Here's how the part is built. I have some questions about the finished solid (model axes, mm). Face numbers are marked on the shaded views. A direction names the side the tool comes from. Give positions to 0.01 mm unless a question says otherwise; leave off trailing zeros. Loops run counter-clockwise (first coordinate to the right, second up) from the corner with the lowest first, then second, coordinate; pieces in that order, holes last.
Q1. Thinking about a two-plate mould opening in X: for the marked faces 1, 2 and 3, which applies, pulls with the +X half, pulls with the -X half, needs draft (parallel to the pull), parting line crosses it, or undercut?
Q2. Suppose I cut it at B-B (x = -24). List the corners of the cut face in (y, z) for me, and give its area (3 significant figures).
Q3. I need wall thicknesses on probe 1 along X at (y, z) = (-11.5, 120); probe 2 along Y at (x, z) = (-76, 101.5); probe 3 along X at (y, z) = (-42.5, 92). Which ranges of each line are inside material? Lowest first, please.
Q4. Suppose I cut it at C-C (y = -19.5). List the corners of the cut face in (x, z) for me.
Q5. Suppose I cut it at A-A (z = 108). List the corners of the cut face in (x, y) for me, and give its area (3 significant figures).
Q6. I'm going to push flat-ended pins straight in: P1, Ø5, axis at x = -58.63, y = 31.73, coming from the +Z side; P2, Ø6, axis at y = -11.5, z = 111.5, coming from the +X side; P3, Ø3.5, axis at y = -46, z = 99.5, coming from the -X side; P4, Ø1.2, axis at x = 14.5, y = 51, coming from the +Z side. Where does each tip first touch, or does it pass through?
Q7. Suppose I cut it at D-D (z = 118). List the corners of the cut face in (x, y) for me, and give its area (3 significant figures).
Q8. For the marked faces 4 and 5, which set-ups out of +Z, -Z, +X, -X, +Y, -Y let a thin tool reach every point of the face, with its end or its side?
```python
from build123d import *

# Parameters (mm, degrees)
SCHIZZO1_W                        = 100.974800609
SCHIZZO1_H                        = 100.97480061
ESTRUSIONE_ESTRUSIONE1_DEPTH      = 3
SCHIZZO3_R                        = 2
TAGLIO_ESTRUSIONE1_DEPTH          = 10
RACCORDO1_R                       = 4
TAGLIO_ESTRUSIONE2_DEPTH          = 3
ESTRUSIONE_ESTRUSIONE2_DEPTH      = 32
ESTRUSIONE_ESTRUSIONE2_DEPTH_BACK = 3
ESTRUSIONE_ESTRUSIONE3_START      = 3
ESTRUSIONE_ESTRUSIONE3_DEPTH      = 3
TAGLIO_ESTRUSIONE3_REACH          = 187.694
SCHIZZO7_W                        = 16.242748833
SCHIZZO7_H                        = 14.432058418
SCHIZZO7_W_2                      = 64.496064987
SCHIZZO7_H_2                      = 15.3
TAGLIO_ESTRUSIONE4_REACH          = 177.413
SCHIZZO8_W                        = 15.4
SCHIZZO8_H                        = 29.105346697
SMUSSO1_SIZE                      = 3
SCHIZZO9_R                        = 2
SCHIZZO9_R_2                      = 1.85551968
TAGLIO_ESTRUSIONE5_DEPTH          = 108.867451135
SCHIZZO10_R                       = 1.6
TAGLIO_ESTRUSIONE6_DEPTH          = 5


with BuildPart() as part:
    # Schizzo1 → Estrusione-Estrusione1 (new body)
    with BuildSketch(Plane(origin=(0, 0, 94.00326253), x_dir=(-1, 0, 0), z_dir=(0, 0, -1))):
        with Locations((31.141269188, 5.2439824)):
            Rectangle(SCHIZZO1_W, SCHIZZO1_H)
    extrude(amount=ESTRUSIONE_ESTRUSIONE1_DEPTH)

    # Schizzo3 → Taglio-Estrusione1 (cut)
    with BuildSketch(Plane.XY.offset(94.00326253)):
        with Locations((-77.128669492, 51.231382705)):
            Circle(SCHIZZO3_R)
        with Locations((14.871330508, 51.231382705)):
            Circle(SCHIZZO3_R)
        with Locations((-77.128669492, -40.768617295)):
            Circle(SCHIZZO3_R)
        with Locations((14.871330508, -40.768617295)):
            Circle(SCHIZZO3_R)
    extrude(amount=-TAGLIO_ESTRUSIONE1_DEPTH, mode=Mode.SUBTRACT)

    # Raccordo1
    raccordo1_edges = [part.edges().sort_by_distance(p)[0] for p in [
        (19.346131117, 55.731382705, 92.50326253),
        (-81.628669492, 55.731382705, 92.50326253),
        (-81.628669492, -45.243417905, 92.50326253),
        (19.346131117, -45.243417905, 92.50326253),
    ]]
    fillet(raccordo1_edges, radius=RACCORDO1_R)

    # Schizzo4 → Taglio-Estrusione2 (cut)
    with BuildSketch(Plane.XY.offset(94.00326253)):
        with BuildLine():
            Line((-74.872857768, -44.07184503), (12.615518783, -44.07184503))
            ThreePointArc((12.615518783, -44.07184503), (12.042903383, -37.940190171), (18.174558242, -38.512805571))
            Line((18.174558242, -38.512805571), (18.174558242, 48.97557098))
            ThreePointArc((18.174558242, 48.97557098), (12.027018614, 48.418930065), (12.652868681, 54.559809829))
            Line((12.652868681, 54.559809829), (-74.910207666, 54.559809829))
            ThreePointArc((-74.910207666, 54.559809829), (-74.300242368, 48.40295558), (-80.457096617, 49.012920878))
            Line((-80.457096617, 49.012920878), (-80.457096617, -38.550155469))
            ThreePointArc((-80.457096617, -38.550155469), (-74.316216853, -37.924305402), (-74.872857768, -44.07184503))
        make_face()
    extrude(amount=-TAGLIO_ESTRUSIONE2_DEPTH, mode=Mode.SUBTRACT)

    # Schizzo5 → Estrusione-Estrusione2 (add, two sides: drawn at the far end of the back side and taken through both)
    with BuildSketch(Plane.XY.offset(94.00326253).offset(-ESTRUSIONE_ESTRUSIONE2_DEPTH_BACK)):
        with BuildLine():
            Line((-77.628669492, 58.731382705), (15.346131117, 58.731382705))
            ThreePointArc((15.346131117, 58.731382705), (20.295878585, 56.681130173), (22.346131117, 51.731382705))
            Line((22.346131117, 51.731382705), (22.346131117, -41.243417905))
            ThreePointArc((22.346131117, -41.243417905), (20.295878585, -46.193165373), (15.346131117, -48.243417905))
            Line((15.346131117, -48.243417905), (-77.628669492, -48.243417905))
            ThreePointArc((-77.628669492, -48.243417905), (-82.578416961, -46.193165373), (-84.628669492, -41.243417905))
            Line((-84.628669492, -41.243417905), (-84.628669492, 51.731382705))
            ThreePointArc((-84.628669492, 51.731382705), (-82.578416961, 56.681130173), (-77.628669492, 58.731382705))
        make_face()
        with BuildLine():
            Line((-77.628669492, 55.731382705), (15.346131117, 55.731382705))
            ThreePointArc((15.346131117, 55.731382705), (18.174558242, 54.559809829), (19.346131117, 51.731382705))
            Line((19.346131117, 51.731382705), (19.346131117, -41.243417905))
            ThreePointArc((19.346131117, -41.243417905), (18.174558242, -44.07184503), (15.346131117, -45.243417905))
            Line((15.346131117, -45.243417905), (-77.628669492, -45.243417905))
            ThreePointArc((-77.628669492, -45.243417905), (-80.457096617, -44.07184503), (-81.628669492, -41.243417905))
            Line((-81.628669492, -41.243417905), (-81.628669492, 51.731382705))
            ThreePointArc((-81.628669492, 51.731382705), (-80.457096617, 54.559809829), (-77.628669492, 55.731382705))
        make_face(mode=Mode.SUBTRACT)
    extrude(amount=ESTRUSIONE_ESTRUSIONE2_DEPTH + ESTRUSIONE_ESTRUSIONE2_DEPTH_BACK)

    # Schizzo6 → Estrusione-Estrusione3 (add)
    with BuildSketch(Plane(origin=(0, 0, 91.00326253), x_dir=(-1, 0, 0), z_dir=(0, 0, -1)).offset(ESTRUSIONE_ESTRUSIONE3_START)):
        with BuildLine():
            Line((-15.346131117, 58.731382705), (77.628669492, 58.731382705))
            ThreePointArc((77.628669492, 58.731382705), (82.578416961, 56.681130173), (84.628669492, 51.731382705))
            Line((84.628669492, 51.731382705), (84.628669492, -41.243417905))
            ThreePointArc((84.628669492, -41.243417905), (82.578416961, -46.193165373), (77.628669492, -48.243417905))
            Line((77.628669492, -48.243417905), (-15.346131117, -48.243417905))
            ThreePointArc((-15.346131117, -48.243417905), (-20.295878585, -46.193165373), (-22.346131117, -41.243417905))
            Line((-22.346131117, -41.243417905), (-22.346131117, 51.731382705))
            ThreePointArc((-22.346131117, 51.731382705), (-20.295878585, 56.681130173), (-15.346131117, 58.731382705))
        make_face()
    extrude(amount=-ESTRUSIONE_ESTRUSIONE3_DEPTH)

    # Schizzo7 → Taglio-Estrusione3 (cut, up to next)
    with BuildSketch(Plane.XZ.offset(48.243417905), mode=Mode.PRIVATE) as taglio_estrusione3_sk1:
        with Locations((2.075800916, 102.505448711)):
            Rectangle(SCHIZZO7_W, SCHIZZO7_H)
    taglio_estrusione3_tool1 = extrude(taglio_estrusione3_sk1.sketch, amount=-TAGLIO_ESTRUSIONE3_REACH, mode=Mode.PRIVATE) & part.part
    # Schizzo7 → Taglio-Estrusione3 (cut, up to next)
    with BuildSketch(Plane.XZ.offset(48.243417905), mode=Mode.PRIVATE) as taglio_estrusione3_sk2:
        with Locations((-40.245307891, 103.027287944)):
            Rectangle(SCHIZZO7_W_2, SCHIZZO7_H_2)
    taglio_estrusione3_tool2 = extrude(taglio_estrusione3_sk2.sketch, amount=-TAGLIO_ESTRUSIONE3_REACH, mode=Mode.PRIVATE) & part.part
    add(taglio_estrusione3_tool1.solids().sort_by_distance((2.075801, -48.243418, 102.505449))[0], mode=Mode.SUBTRACT)
    add(taglio_estrusione3_tool2.solids().sort_by_distance((-40.245308, -48.243418, 103.027288))[0], mode=Mode.SUBTRACT)

    # Schizzo8 → Taglio-Estrusione4 (cut, up to next)
    with BuildSketch(Plane(origin=(22.346131117, 0, 0), x_dir=(0, 0, -1), z_dir=(1, 0, 0)), mode=Mode.PRIVATE) as taglio_estrusione4_sk1:
        with Locations((-106.101551061, -6.264379468)):
            Rectangle(SCHIZZO8_W, SCHIZZO8_H)
    taglio_estrusione4_tool1 = extrude(taglio_estrusione4_sk1.sketch, amount=-TAGLIO_ESTRUSIONE4_REACH, mode=Mode.PRIVATE) & part.part
    add(taglio_estrusione4_tool1.solids().sort_by_distance((22.346131, -6.264379, 106.101551))[0], mode=Mode.SUBTRACT)

    # Smusso1
    smusso1_edges = [part.edges().sort_by_distance(p)[0] for p in [
        (2.075800916, -48.243417905, 95.289419502),
    ]]
    chamfer(smusso1_edges, length=SMUSSO1_SIZE - 0.0001)  # a hair under: the kernel refuses the full size

    # Schizzo9 → Taglio-Estrusione5 (cut, through all)
    with BuildSketch(Plane.XY.offset(94.00326253)):
        with Locations((-77.128669492, 51.231382705)):
            Circle(SCHIZZO9_R)
        with Locations((14.871330508, 51.231382705)):
            Circle(SCHIZZO9_R_2)
        with Locations((14.871330508, -40.768617295)):
            Circle(SCHIZZO9_R)
        with Locations((-77.128669492, -40.768617295)):
            Circle(SCHIZZO9_R)
    extrude(amount=-TAGLIO_ESTRUSIONE5_DEPTH, mode=Mode.SUBTRACT)

    # Schizzo10 → Taglio-Estrusione6 (cut)
    with BuildSketch(Plane(origin=(0, 0, 88.00326253), x_dir=(-1, 0, 0), z_dir=(0, 0, -1))):
        with Locations((3.653868883, 31.731382705)):
            Circle(SCHIZZO10_R)
        with Locations((3.653868883, -14.268617295)):
            Circle(SCHIZZO10_R)
        with Locations((58.628669492, -14.268617295)):
            Circle(SCHIZZO10_R)
        with Locations((58.628669492, 31.731382705)):
            Circle(SCHIZZO10_R)
    extrude(amount=-TAGLIO_ESTRUSIONE6_DEPTH, mode=Mode.SUBTRACT)


solid = part.part
```
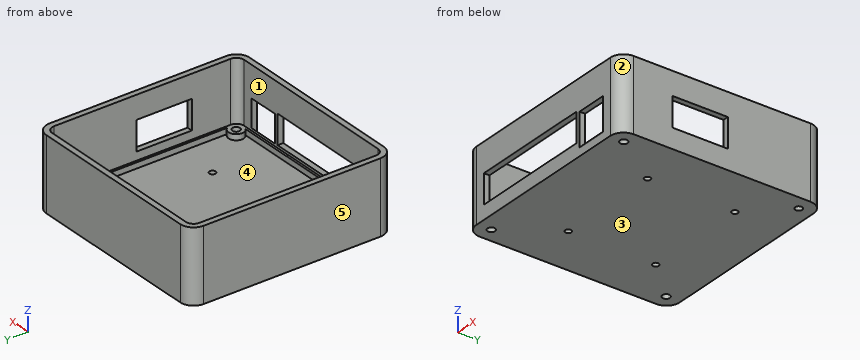
Solutions:
1. face 1: undercut
1. face 2: pulls with the +X half
1. face 3: needs draft
2. outline: (-48.24, 88) - (58.73, 88) - (58.73, 126) - (55.73, 126) - (55.73, 94) - (54.56, 94) - (54.56, 91) - (-44.07, 91) - (-44.07, 94) - (-45.24, 94) - (-45.24, 95.38) - (-48.24, 95.38) - close; (-48.24, 110.68) - (-45.24, 110.68) - (-45.24, 126) - (-48.24, 126) - close
2. area: 492 mm2
3. probe 1: x = -84.63 to -81.63, 19.35 to 22.35
3. probe 2: y = -48.24 to -45.24, 55.73 to 58.73
3. probe 3: x = -84.51 to -78.13, -76.13 to -73.52, 11.27 to 13.87, 15.87 to 22.23
4. outline: (-84.63, 88) - (22.35, 88) - (22.35, 98.4) - (19.35, 98.4) - (19.35, 94) - (18.17, 94) - (18.17, 91) - (-80.46, 91) - (-80.46, 94) - (-81.63, 94) - (-81.63, 126) - (-84.63, 126) - close; (19.35, 113.8) - (22.35, 113.8) - (22.35, 126) - (19.35, 126) - close
5. outline: (-84.63, -41.24) arc R7 ccw to (-77.63, -48.24) - (-72.49, -48.24) - (-72.49, -45.24) - (-77.63, -45.24) arc R4 cw to (-81.63, -41.24) - (-81.63, 51.73) arc R4 cw to (-77.63, 55.73) - (15.35, 55.73) arc R4 cw to (19.35, 51.73) - (19.35, 8.29) - (22.35, 8.29) - (22.35, 51.73) arc R7 ccw to (15.35, 58.73) - (-77.63, 58.73) arc R7 ccw to (-84.63, 51.73) - close; (-8, -48.24) - (-6.05, -48.24) - (-6.05, -45.24) - (-8, -45.24) - close; (10.2, -48.24) - (15.35, -48.24) arc R7 ccw to (22.35, -41.24) - (22.35, -20.82) - (19.35, -20.82) - (19.35, -41.24) arc R4 cw to (15.35, -45.24) - (10.2, -45.24) - close
5. area: 890 mm2
6. P1: stops at z = 91
6. P2: stops at x = 22.35
6. P3: stops at x = -83.95
6. P4: passes through
7. outline: (-84.63, -41.24) arc R7 ccw to (-77.63, -48.24) - (15.35, -48.24) arc R7 ccw to (22.35, -41.24) - (22.35, 51.73) arc R7 ccw to (15.35, 58.73) - (-77.63, 58.73) arc R7 ccw to (-84.63, 51.73) - close; hole (-81.63, -41.24) arc R4 ccw to (-77.63, -45.24) - (15.35, -45.24) arc R4 ccw to (19.35, -41.24) - (19.35, 51.73) arc R4 ccw to (15.35, 55.73) - (-77.63, 55.73) arc R4 ccw to (-81.63, 51.73) - close
7. area: 1,220 mm2
8. face 4: +Z
8. face 5: +Z, -Z, -X, +Y, -Y
